For this review, take the finished solid that the model builds, in its own axes (mm). A direction names the side the tool comes from. Round coordinates to 2 decimals unless told otherwise and drop trailing zeros. Write each loop counter-clockwise with the first axis right and the second up, starting at its lowest first coordinate (ties: lowest second). Pieces come first, ordered by that corner, then holes. Notation, with made-up numbers: (20.5, 88) -> (39.5, 88) arc R13 cw to (39.5, 100) -> close; hole circle Ø4 at (-26, 13). An arc over 180 degrees is marked (long way). Answer as CSV lines item,"result". Start each with the question number.
Item 1: Machinability: for faces 1 (the flat face through (131, 63, 118)), 2 (the flat face through (138.04, -19.72, -10.76)), 3 (the flat face through (173, -40, 28)), 4 (the flat face through (138.28, -18.2, -7.77)), 5 (the flat face through (-80, 3, 75)), which of the approach directions +Z, -Z, +X, -X, +Y, -Y give a long, thin tool a straight path to every point of the face, cutting with its end or side? Answer none if there is none.
Item 2: Take a section at D-D on z = -107.5. Give the boundary of the cut face in (x, y).
Item 3: Mouldability with a two-part tool opening along X and no side actions: class faces 6 (the flat face through (-82, 0, 77)), 7 (the cylindrical face through (101.2, -18.2, 19.18)), 8 (the flat face through (125.907, -19.72, 60.171)) as +X half, -X half, draft (parallel to the pull), parting line (faces both ways), or undercut.
Item 4: Take a section at C-C on z = 19. Give the boundary of the cut face in (x, y).
Item 5: For pin 1 Ø5 at (y, z) = (43.5, -124.5) entering from +X; pin 2 Ø1 at (x, z) = (-126, 87) entering from -Y; pin 3 Ø8 at (x, y) = (96, -16.5) entering from +Z, all flat-tipped, find the tip position at first contact; note any pin that passes through.
Item 6: Wall thickness on probe 1 along X at (y, z) = (33, 0); probe 2 along X at (y, z) = (-12.5, 0): over which ranges is each line inside the solid? List them lowest first. Write a range as from..to.
Item 7: Take a section at B-B on y = -22. Give the boundary of the cut face in (x, z), then the cut area to 3 significant figures.
Item 8: Take a section at A-A on x = 0. Give the boundary of the cut face in (y, z).
```python
from build123d import *

# Parameters (mm, degrees)
SKETCH2_R                 = 178
SKETCH2_R_2               = 100
BOSS_EXTRUDE1_DEPTH       = 3
SKETCH3_R                 = 178
SKETCH3_R_2               = 175
BOSS_EXTRUDE2_DEPTH       = 60
CUT_EXTRUDE2_DEPTH        = 25
BOSS_EXTRUDE17_DEPTH      = 40
BOSS_EXTRUDE17_DEPTH_BACK = 3


with BuildPart() as part:
    # Sketch2 → Boss-Extrude1 (new body)
    with BuildSketch(Plane(origin=(0, 0, 0), x_dir=(1, 0, 0), z_dir=(0, 1, 0))):
        Circle(SKETCH2_R)
        Circle(SKETCH2_R_2, mode=Mode.SUBTRACT)
    extrude(amount=BOSS_EXTRUDE1_DEPTH)

    # Sketch3 → Boss-Extrude2 (add)
    with BuildSketch(Plane(origin=(0, 3, 0), x_dir=(1, 0, 0), z_dir=(0, 1, 0))):
        Circle(SKETCH3_R)
        Circle(SKETCH3_R_2, mode=Mode.SUBTRACT)
    extrude(amount=BOSS_EXTRUDE2_DEPTH)

    # Sketch5 → Cut-Extrude2 (cut)
    with BuildSketch(Plane(origin=(0, 3, 0), x_dir=(1, 0, 0), z_dir=(0, 1, 0))):
        with BuildLine():
            Line((174.470835958, 13.59880142), (99.697620548, 7.770743669))
            ThreePointArc((99.697620548, 7.770743669), (99.924376542, 3.888312311), (100, 0))
            ThreePointArc((100, 0), (97.525905257, -22.106510438), (90.226043925, -43.11914885))
            Line((90.226043925, -43.11914885), (157.895576869, -75.458510488))
            ThreePointArc((157.895576869, -75.458510488), (170.6703342, -38.686393266), (175, 0))
            ThreePointArc((175, 0), (174.867658949, 6.804546543), (174.470835958, 13.59880142))
        make_face()
    extrude(amount=-CUT_EXTRUDE2_DEPTH, mode=Mode.SUBTRACT)

    # Sketch16 → Boss-Extrude17 (add, two sides)
    with BuildSketch(Plane.XZ) as boss_extrude17_sk:
        with BuildLine():
            Line((160.602358187, 76.752084954), (90.226043925, 43.11914885))
            ThreePointArc((90.226043925, 43.11914885), (98.311722962, 18.29768095), (99.697620548, -7.770743669))
            Line((99.697620548, -7.770743669), (177.461764575, -13.83192373))
            ThreePointArc((177.461764575, -13.83192373), (174.994866873, 32.569872091), (160.602358187, 76.752084954))
        make_face()
        with BuildLine():
            Line((159.165948647, 72.740640575), (94.186972199, 41.687099538))
            ThreePointArc((94.186972199, 41.687099538), (101.261074651, 18.846611379), (102.878105019, -5.009541657))
            Line((102.878105019, -5.009541657), (174.678319853, -10.605874466))
            ThreePointArc((174.678319853, -10.605874466), (172.045515184, 32.020941663), (159.165948647, 72.740640575))
        make_face(mode=Mode.SUBTRACT)
    extrude(amount=BOSS_EXTRUDE17_DEPTH)
    extrude(boss_extrude17_sk.sketch, amount=-BOSS_EXTRUDE17_DEPTH_BACK)


solid = part.part
```
Output values:
1,face 1,"+Z, -Z, +X, -X, +Y"
1,face 2,"-Z, -X, -Y"
1,face 3,"+Z, -Z, +X, -X, -Y"
1,face 4,"+Y, -Y"
1,face 5,"+Y"
2,outline,"(-141.87, 0) -> (141.87, 0) -> (141.87, 63) -> (138.09, 63) -> (138.09, 3) -> (-138.09, 3) -> (-138.09, 63) -> (-141.87, 63) -> close"
3,face 6,"draft"
3,face 7,"undercut"
3,face 8,"-X half"
4,outline,"(-176.98, 0) -> (-98.18, 0) -> (-98.18, 3) -> (-173.97, 3) -> (-173.97, 63) -> (-176.98, 63) -> close; (98.18, -40) -> (101.23, -40) -> (101.23, 3) -> (98.18, 3) -> close; (173.97, -40) -> (176.98, -40) -> (176.98, 63) -> (173.97, 63) -> close"
5,pin 1,"stops at x = 129.61"
5,pin 2,"stops at y = 0"
5,pin 3,"stops at z = 47.79"
6,probe 1,"x = -178..-175, 175..178"
6,probe 2,"x = 100..103, 175..178"
7,outline,"(90.23, 43.12) arc R100 cw to (99.7, -7.77) -> (177.46, -13.83) arc R178 ccw to (160.6, 76.75) -> close; hole (94.19, 41.69) arc R103 cw to (102.88, -5.01) -> (174.68, -10.61) arc R175 ccw to (159.17, 72.74) -> close"
7,area,"869 mm^2"
8,outline,"(0, -178) -> (63, -178) -> (63, -175) -> (3, -175) -> (3, -100) -> (0, -100) -> close; (0, 100) -> (3, 100) -> (3, 175) -> (63, 175) -> (63, 178) -> (0, 178) -> close"
